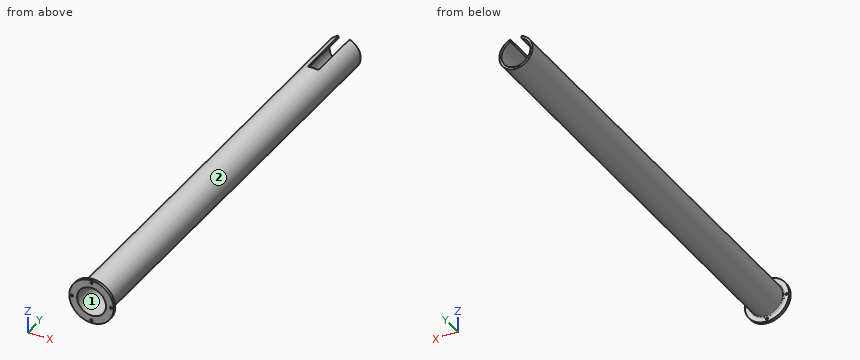
```python
from build123d import *
from build123d.topology import SkipClean

# Parameters (mm, degrees)
SKETCH1_R           = 30
SKETCH1_R_2         = 26
BOSS_EXTRUDE1_DEPTH = 800
BOSS_EXTRUDE2_START = 5
SKETCH2_R           = 40
SKETCH2_R_2         = 26
SKETCH2_R_3         = 2
BOSS_EXTRUDE2_DEPTH = 5
FILLET1_R           = 2
SKETCH3_W           = 20
SKETCH3_H           = 53.092169015
CUT_EXTRUDE1_DEPTH  = 100
FILLET2_R           = 5


with BuildPart() as part:
    # Sketch1 → Boss-Extrude1 (new body)
    with BuildSketch(Plane(origin=(0, 0, 0), x_dir=(1, 0, 0), z_dir=(0, 1, 0))):
        with Locations(Location((0, 0, 0), (0, 0, 270))):
            Circle(SKETCH1_R)
        with Locations(Location((0, 0, 0), (0, 0, 270))):
            Circle(SKETCH1_R_2, mode=Mode.SUBTRACT)
    extrude(amount=BOSS_EXTRUDE1_DEPTH)

    # Sketch2 → Boss-Extrude2 (add)
    with SkipClean():  # the faces are left unmerged after this step: merging them gives an invalid solid
        with BuildSketch(Plane.XZ.offset(BOSS_EXTRUDE2_START)):
            with Locations(Location((0, 0, 0), (0, 0, 270))):
                Circle(SKETCH2_R)
            with Locations(Location((0, 0, 0), (0, 0, 270))):
                Circle(SKETCH2_R_2, mode=Mode.SUBTRACT)
            with Locations(Location((0, 35, 0), (0, 0, 270))):
                Circle(SKETCH2_R_3, mode=Mode.SUBTRACT)
            with Locations(Location((35, 0, 0), (0, 0, 270))):
                Circle(SKETCH2_R_3, mode=Mode.SUBTRACT)
            with Locations(Location((-35, 0, 0), (0, 0, 270))):
                Circle(SKETCH2_R_3, mode=Mode.SUBTRACT)
            with Locations(Location((0, -35, 0), (0, 0, 270))):
                Circle(SKETCH2_R_3, mode=Mode.SUBTRACT)
        extrude(amount=-BOSS_EXTRUDE2_DEPTH)

    # Fillet1
    fillet1_edges = [part.edges().sort_by_distance(p)[0] for p in [
        (0, 0, -30),
    ]]
    fillet(fillet1_edges, radius=FILLET1_R)

    # Sketch3 → Cut-Extrude1 (cut)
    with SkipClean():  # the faces are left unmerged after this step: merging them gives an invalid solid
        with BuildSketch(Plane(origin=(0, 800, 0), x_dir=(1, 0, 0), z_dir=(0, 1, 0))):
            with Locations((0, -32.696174879)):
                Rectangle(SKETCH3_W, SKETCH3_H)
        extrude(amount=-CUT_EXTRUDE1_DEPTH, mode=Mode.SUBTRACT)

    # Fillet2
    fillet2_edges = [part.edges().sort_by_distance(p)[0] for p in [
        (10, 700, 26.142135624),
        (-10, 700, 26.142135624),
    ]]
    fillet(fillet2_edges, radius=FILLET2_R)


solid = part.part
```
Check sheet for the modelled part. Datum: model origin and axes. Units: mm. Face numbers are marked on the shaded views. Give positions to 0.01 mm unless a question says otherwise; leave off trailing zeros. Order: outer loops, then holes, each group sorted by start corner. A loop starts at its lowest first (then second) coordinate and runs counter-clockwise, first axis right, second up. Notation, with made-up numbers: M 36.25,77.25 L 85.25,77.25 A10 cw 85.25,94.25 Z; hole C 81,50 d6. An arc over 180 degrees is marked long. Answer in a Markdown table with one row per item. Add a question column.
Q1. Thickness scan on L1, parallel to X at y = -2.8, z = 0; L2, parallel to X at y = 526, z = -1. Record the ranges inside material, lowest first.
Q2. Sectioned sample at A-A, the plane y = 263. Record the boundary of the cut face in (x, z).
Q3. Gauge pin test, flat ends, axial feed: pin 1 Ø6 at (y, z) = (481, 9) entering from +X; pin 2 Ø2 at (x, z) = (0.5, 28) entering from +Y; pin 3 Ø5 at (x, y) = (-29.5, 661) entering from -Z; pin 4 Ø5 at (x, z) = (-11.5, 22.5) entering from -Y. Record the tip position at first contact, or that the pin passes through.
Q4. Sectioned sample at B-B, the plane y = 739. Record the boundary of the cut face in (x, z).
Q5. Release check for a two-part mould opening along Z. For the marked faces 1 and 2 record: released by +Z, released by -Z, zero draft, split by the parting line, or undercut.
Verdict:
| question | item | result |
|---|---|---|
| 1 | L1 | -40 to -37, -33 to -26, 26 to 33, 37 to 40 |
| 1 | L2 | -29.98 to -25.98, 25.98 to 29.98 |
| 2 | outline | C 0,0 d60; hole C 0,0 d52 |
| 3 | pin 1 | x = 29.39 |
| 3 | pin 2 | y = 700 |
| 3 | pin 3 | z = -13.08 |
| 3 | pin 4 | y = -5 |
| 4 | outline | M -10,24 L -10,28.28 A30 ccw long 10,28.28 L 10,24 A26 cw long Z |
| 5 | face 1 | undercut |
| 5 | face 2 | split by the parting line |
